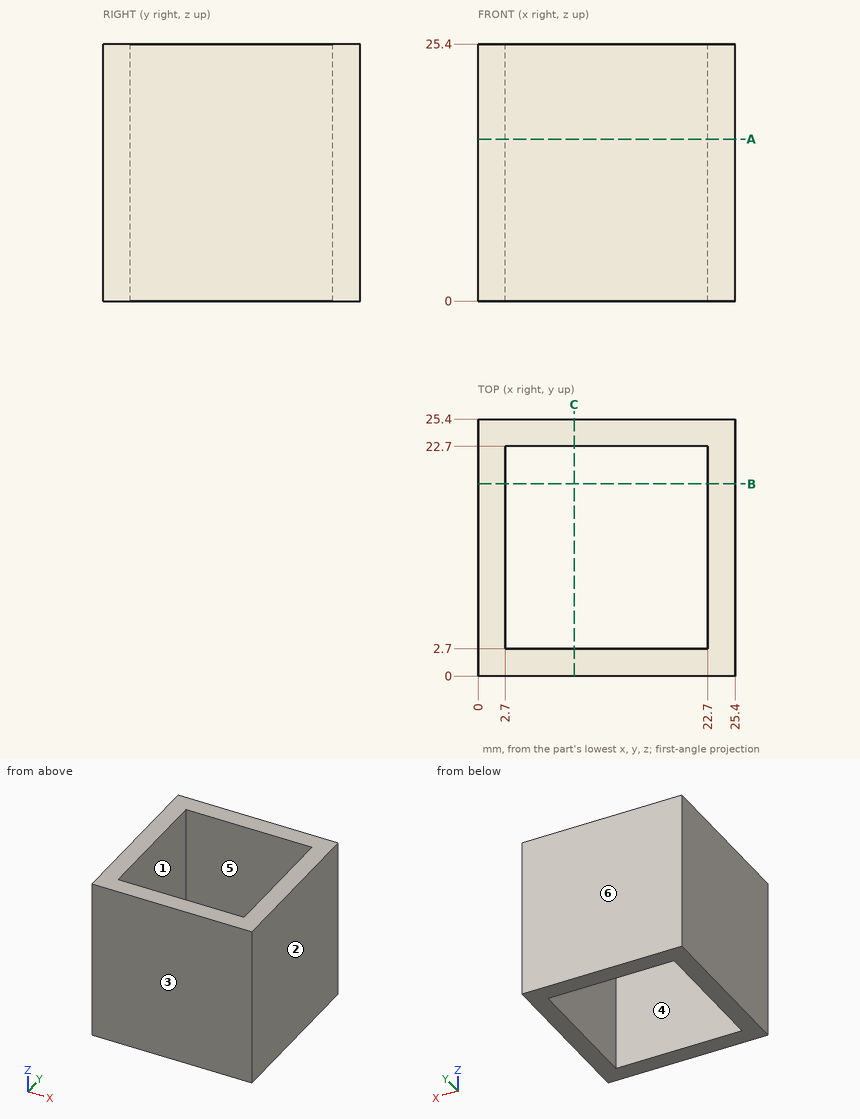
Check sheet for the drawn part. Datum: minimum x, y, z corner. Units: mm. A direction names the side the tool comes from. Give positions to 0.01 mm unless a question says otherwise; leave off trailing zeros. Write each loop counter-clockwise with the first axis right and the second up, starting at its lowest first coordinate (ties: lowest second). Pieces come first, ordered by that corner, then holes. Notation, with made-up numbers: M 13,-20 L 68,-20 A19 cw 68,6 Z; hole C 42,31 d7. An arc over 180 degrees is marked long. One line per question, with ' | ' between items.
1. Cross-section at B-B (y = 19). Enter the section's corners in (x, z).
Ans:
outline: M 0,0 L 2.7,0 L 2.7,25.4 L 0,25.4 Z; M 22.7,0 L 25.4,0 L 25.4,25.4 L 22.7,25.4 Z
2. Cross-section at A-A (z = 16). Enter the section's corners in (x, y).
Ans:
outline: M 0,0 L 25.4,0 L 25.4,25.4 L 0,25.4 Z; hole M 2.7,2.7 L 22.7,2.7 L 22.7,22.7 L 2.7,22.7 Z
3. Set-up check for the marked faces 5 and 6: record each of +Z, -Z, +X, -X, +Y, -Y from which the full face is reachable in a straight line by a thin tool's end or side.
Ans:
face 5: +Z, -Z | face 6: +Z, -Z, +X, -X, +Y
4. Scan line: line 1 along Y through (x, z) = (18.75, 23.5). Record every from-to range of solid material in increasing order. Write a range as from..to.
Ans:
line 1: 0..2.7, 22.7..25.4
5. Mould release check, pull along Y, two halves, no side actions. Record for the marked faces 1, 2, 3 and 4: released by +Y, released by -Y, zero draft, split by the parting line, or undercut.
Ans:
face 1: undercut | face 2: zero draft | face 3: released by -Y | face 4: undercut
